The listing builds one solid part. Answer for the finished solid, in the listing's coordinates (mm). Face numbers are marked on the shaded views. A direction names the side the tool comes from. Round coordinates to 2 decimals unless told otherwise and drop trailing zeros. Order: outer loops, then holes, each group sorted by start corner. A loop starts at its lowest first (then second) coordinate and runs counter-clockwise, first axis right, second up. Notation, with made-up numbers: (82, 82) -> (118, 82) arc R20 ccw to (118, 98) -> close; hole circle Ø10 at (40.5, 70.25). An arc over 180 degrees is marked (long way). Return JSON: item names as keys, results as strings. Group by question number.
(1) The part is cut by section D-D (x = -24.5). Determine the outline of the cut face in (y, z).
(2) Which of the six approach directions +Z, -Z, +X, -X, +Y, -Y give full straight-line access (tool end or side, diameter ignored) to the marked faces 4, 5 and 6?
(3) The part is cut by section A-A (y = -9). Determine the outline of the cut face in (x, z).
(4) The part is cut by section B-B (y = 16). Determine the outline of the cut face in (x, z).
(5) Each of these flat-tipped pins is pushed along its axis until it touches: pin 1 (2 mm diameter, centred on x = -25.5, z = -4.5, fed in from -Y); pin 2 (6 mm diameter, centred on y = -14.5, z = -2.5, fed in from +X); pin 3 (4.5 mm diameter, centred on x = -24.52, y = 10, fed in from -Z); pin 4 (11 mm diameter, centred on x = 39.5, y = 8.5, fed in from +Z). Where does it stop, or does it pass through?
(6) The part is cut by section C-C (z = -4.75). Count the separate pieces of the cut face and the enclosed holes in it, plus the area to 3 significant figures.
(7) Consider line 1 (Y direction, x = 59.5, z = -2); line 2 (Y direction, x = 44, z = -5.25); line 3 (Z direction, x = -0.5, y = -7.5). Determine where each line is inside the solid, lowest interval first. Write a range as [from, to].
(8) Determine the mould class of the marked faces 1, 2 and 3 for opening direction X: +X half, -X half, draft (parallel to the pull), parting line (faces both ways), or undercut.
from build123d import *

# Parameters (mm, degrees)
BOSS_EXTRUDE1_DEPTH = 20
EXTRUDE_THIN3_DEPTH = 21
SKETCH3_R           = 2.75
CUT_EXTRUDE1_DEPTH  = 73.35515227
FILLET2_R           = 3
SKETCH4_R           = 1.25
CUT_EXTRUDE2_DEPTH  = 10


with BuildPart() as part:
    # Sketch1 → Boss-Extrude1 (new body)
    with BuildSketch(Plane(origin=(0, 0, 0), x_dir=(1, 0, 0), z_dir=(0, 1, 0))):
        Polygon((-32.516534914, -1.83981797), (-32.516534914, 13.66018203), (67.483465086, 13.66018203), (67.483465086, -1.83981797), (50.983465086, -1.83981797), (50.983465086, 1.63642231), (50.983465086, 6.16018203), (48.983465086, 6.16018203), (48.983465086, 0.16018203), (34.983465086, 0.16018203), (34.983465086, 6.16018203), (32.983465086, 6.16018203), (32.983465086, 1.63642231), (32.983465086, -1.83981797), (1.983465086, -1.83981797), (1.983465086, 1.63642231), (1.983465086, 6.16018203), (-0.016534914, 6.16018203), (-0.016534914, 0.16018203), (-14.016534914, 0.16018203), (-14.016534914, 6.16018203), (-16.016534914, 6.16018203), (-16.016534914, 1.63642231), (-16.016534914, -1.83981797), align=None)
    extrude(amount=BOSS_EXTRUDE1_DEPTH)

    # Sketch2 → Extrude-Thin3 (add)
    with BuildSketch(Plane.XZ):
        Polygon((-19.016534914, 1.83981797), (-19.016534914, -13.66018203), (4.983465086, -13.66018203), (4.983465086, 1.83981797), (1.983465086, 1.83981797), (1.983465086, -10.66018203), (-16.016534914, -10.66018203), (-16.016534914, 1.83981797), align=None)
        Polygon((50.983465086, 1.83981797), (50.983465086, -10.66018203), (32.983465086, -10.66018203), (32.983465086, 1.83981797), (29.983465086, 1.83981797), (29.983465086, -13.66018203), (53.983465086, -13.66018203), (53.983465086, 1.83981797), align=None)
    extrude(amount=EXTRUDE_THIN3_DEPTH)

    # Sketch3 → Cut-Extrude1 (cut, through all)
    with BuildSketch(Plane(origin=(0, 0, -13.66018203), x_dir=(-1, 0, 0), z_dir=(0, 0, -1))):
        with Locations((24.516534914, 10)):
            Circle(SKETCH3_R)
        with Locations((-59.483465086, 10)):
            Circle(SKETCH3_R)
        with Locations((-17.483465086, 10)):
            Circle(SKETCH3_R)
    extrude(amount=-CUT_EXTRUDE1_DEPTH, mode=Mode.SUBTRACT)

    # Fillet2
    fillet2_edges = [part.edges().sort_by_distance(p)[0] for p in [
        (17.483465086, 0, -13.66018203),
        (29.983465086, -10.5, -13.66018203),
        (53.983465086, -10.5, -13.66018203),
        (60.733465086, 0, -13.66018203),
        (67.483465086, 0, -5.91018203),
        (67.483465086, 10, -13.66018203),
        (67.483465086, 20, -5.91018203),
        (17.483465086, 20, -13.66018203),
        (-32.516534914, 20, -5.91018203),
        (-32.516534914, 0, -5.91018203),
        (-19.016534914, 0, -5.91018203),
        (4.983465086, -10.5, -13.66018203),
        (-19.016534914, -10.5, -13.66018203),
        (-25.766534914, 0, -13.66018203),
        (-32.516534914, 10, -13.66018203),
        (53.983465086, 0, -5.91018203),
    ]]
    fillet(fillet2_edges, radius=FILLET2_R)

    # Sketch4 → Cut-Extrude2 (cut)
    with BuildSketch(Plane(origin=(0, 0, -13.66018203), x_dir=(-1, 0, 0), z_dir=(0, 0, -1))):
        with Locations((2.516534914, -9)):
            Circle(SKETCH4_R)
        with Locations((11.516534914, -9)):
            Circle(SKETCH4_R)
    extrude(amount=-CUT_EXTRUDE2_DEPTH, mode=Mode.SUBTRACT)


solid = part.part
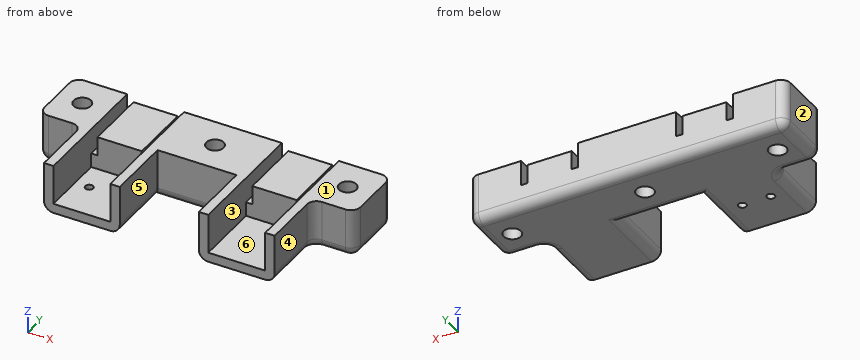
Answer below:
{
 "1": {"outline": "(0, -10.66) arc R3 ccw to (3, -13.66) -> (7.25, -13.66) -> (7.25, 1.84) -> (0, 1.84) -> close; (12.75, -13.66) -> (17, -13.66) arc R3 ccw to (20, -10.66) -> (20, 1.84) -> (12.75, 1.84) -> close"},
 "2": {"face 4": "+Z, -Z, +X, -Y", "face 5": "+Z, -Z, -Y", "face 6": "+Z, -Y"},
 "3": {"outline": "(-19.02, -10.66) arc R3 ccw to (-16.02, -13.66) -> (-12.77, -13.66) -> (-12.77, -10.66) -> (-16.02, -10.66) -> (-16.02, 1.84) -> (-19.02, 1.84) -> close; (-10.27, -13.66) -> (-3.77, -13.66) -> (-3.77, -10.66) -> (-10.27, -10.66) -> close; (-1.27, -13.66) -> (1.98, -13.66) arc R3 ccw to (4.98, -10.66) -> (4.98, 1.84) -> (1.98, 1.84) -> (1.98, -10.66) -> (-1.27, -10.66) -> close; (29.98, -10.66) arc R3 ccw to (32.98, -13.66) -> (50.98, -13.66) arc R3 ccw to (53.98, -10.66) -> (53.98, 1.84) -> (50.98, 1.84) -> (50.98, -10.66) -> (32.98, -10.66) -> (32.98, 1.84) -> (29.98, 1.84) -> close"},
 "4": {"outline": "(-32.52, -10.66) arc R3 ccw to (-29.52, -13.66) -> (64.48, -13.66) arc R3 ccw to (67.48, -10.66) -> (67.48, 1.84) -> (50.98, 1.84) -> (50.98, -6.16) -> (48.98, -6.16) -> (48.98, -0.16) -> (34.98, -0.16) -> (34.98, -6.16) -> (32.98, -6.16) -> (32.98, 1.84) -> (1.98, 1.84) -> (1.98, -6.16) -> (-0.02, -6.16) -> (-0.02, -0.16) -> (-14.02, -0.16) -> (-14.02, -6.16) -> (-16.02, -6.16) -> (-16.02, 1.84) -> (-32.52, 1.84) -> close"},
 "5": {"pin 1": "stops at y = 0", "pin 2": "stops at x = 53.98", "pin 3": "passes through", "pin 4": "stops at z = -0.16"},
 "6": {"separate pieces": "5", "enclosed holes": "3", "area": "2,020 mm²"},
 "7": {"line 1": "y = [0, 7.25], [12.75, 20]", "line 2": "y = [0, 20]", "line 3": "z = [-13.66, -10.66]"},
 "8": {"face 1": "draft", "face 2": "-X half", "face 3": "undercut"}
}
